Geometry check sheet. Reference: the model listing, model coordinates, mm. Round coordinates to 2 decimals unless told otherwise and drop trailing zeros. Loops run counter-clockwise (first coordinate to the right, second up) from the corner with the lowest first, then second, coordinate; pieces in that order, holes last. Notation, with made-up numbers: M 50.5,39 L 59.5,39 A19 ccw 59.5,44 Z; hole C -1,61 d3. An arc over 180 degrees is marked long. Use one line per item in the form item = value. Start each with the question number.
1. Material ranges on line 1 (Y direction, x = 57.5, z = 4.75); line 2 (Z direction, x = -132.5, y = 249); line 3 (X direction, y = 39, z = 4.5), recorded low to high.
2. Cross-section at B-B (z = 4). Record the boundary of the cut face in (x, y).
3. Cross-section at C-C (x = -11). Record the boundary of the cut face in (y, z), then the cut area to 3 significant figures.
4. Cross-section at A-A (y = 167). Record the boundary of the cut face in (x, z).
5. Go/stop test with flat-tipped pins: pin 1 (5 mm diameter, centred on y = 164.5, z = -3.5, fed in from -X); pin 2 (10 mm diameter, centred on y = 216, z = -4, fed in from -X); pin 3 (10 mm diameter, centred on x = -13, z = -3, fed in from -Y). Record where each tip stops, or that it passes through.
6. Cross-section at D-D (y = 114). Record the boundary of the cut face in (x, z).
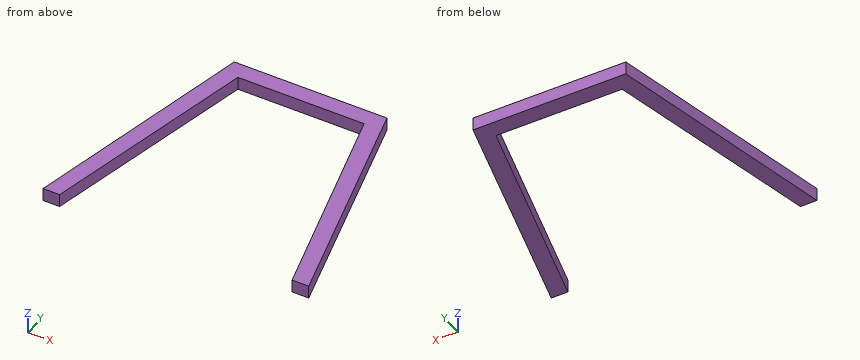
```python
from build123d import *

# Parameters (mm, degrees)
A_FRAME_BLANK_DEPTH   = 10
HOLLOW_WALL_2MM_START = -8
HOLLOW_WALL_2MM_DEPTH = 16


# Read off the part's stored shape, not the designer's step: Hollow_Wall_2mm
with BuildPart() as part:
    # A_Frame_Profile → A_Frame_Blank (new, symmetric)
    with BuildSketch(Plane.XY):
        Polygon((-200, 0), (-115, 350), (115, 350), (200, 0), (175, 0), (95, 325), (-95, 325), (-175, 0), align=None)
    extrude(amount=A_FRAME_BLANK_DEPTH, both=True)

    # Hollow_Wall_2mm outline → Hollow_Wall_2mm (cut)
    with BuildSketch(Plane.XY.offset(HOLLOW_WALL_2MM_START)):
        Polygon((-197.456151033, 2), (-176.567392981, 2), (-96.567392981, 327), (96.567392981, 327), (176.567392981, 2), (197.456151033, 2), (113.427579604, 348), (-113.427579604, 348), align=None)
    extrude(amount=HOLLOW_WALL_2MM_DEPTH, mode=Mode.SUBTRACT)


solid = part.part
```
Reported:
q1.line_1 = 325 to 327, 348 to 350
q1.line_2 = -10 to -8, 8 to 10
q1.line_3 = -190.53 to -188.47, -167.46 to -165.4, 165.4 to 167.46, 188.47 to 190.53
q2.outline = M -200,0 L -175,0 L -95,325 L 95,325 L 175,0 L 200,0 L 115,350 L -115,350 Z; hole M -197.46,2 L -176.57,2 L -96.57,327 L 96.57,327 L 176.57,2 L 197.46,2 L 113.43,348 L -113.43,348 Z
q3.outline = M 325,-10 L 350,-10 L 350,10 L 325,10 Z; hole M 327,-8 L 348,-8 L 348,8 L 327,8 Z
q3.area = 164 mm²
q4.outline = M -159.44,-10 L -133.89,-10 L -133.89,10 L -159.44,10 Z; M 133.89,-10 L 159.44,-10 L 159.44,10 L 133.89,10 Z; hole M -157.38,-8 L -135.95,-8 L -135.95,8 L -157.38,8 Z; hole M 135.95,-8 L 157.38,-8 L 157.38,8 L 135.95,8 Z
q5.pin_1 = -160.66
q5.pin_2 = -148.76
q5.pin_3 = 325
q6.outline = M -172.31,-10 L -146.94,-10 L -146.94,10 L -172.31,10 Z; M 146.94,-10 L 172.31,-10 L 172.31,10 L 146.94,10 Z; hole M -170.26,-8 L -149,-8 L -149,8 L -170.26,8 Z; hole M 149,-8 L 170.26,-8 L 170.26,8 L 149,8 Z
